Autodesk Inventor part; units mm, degrees
ref_plane "작업 평면1" through (-0.2823, -5.2823, -2.8) normal (0, 0, -1) x (0, 1, 0)
ref_plane "작업 평면2" through (1.8306, -3.1694, -7.8) normal (0, 0, -1) x (0, 1, 0)
ref_plane "YZ Plane" through (0, 0, 0) normal (1, 0, 0) x (0, 1, 0)
sketch "스케치1" plane through (0, 0, 0) normal (0, 0, 1) x (1, 0, 0)
  line L0 (5, 1.4434) -> (6.25, 0.7217)
  line L1 (6.25, 0.7217) -> (6.25, -0.7217)
  line L2 (6.25, -0.7217) -> (5, -1.4434)
  line L3 (5, -1.4434) -> (3.75, -0.7217)
  line L4 (3.75, -0.7217) -> (3.75, 0.7217)
  line L5 (3.75, 0.7217) -> (5, 1.4434)
  circle A0 centre (5, 0) radius 5
  circle A1 centre (5, 0) radius 5
  point P0 (0, 0)
ref_plane "작업 평면1" through (-0.2823, -5.2823, -2.8) normal (0, 0, -1) x (0, 1, 0)
extrude "돌출1" add sketch "스케치1" against normal up to surface (2.8 mm away)
sketch "스케치2" plane through (5, 0, -2.8) normal (0, 0, -1) x (-1, 0, 0)
  circle A0 centre (0, 0) radius 3
  circle A1 centre (0, 0) radius 2
  point P0 (5, 0)
ref_plane "작업 평면2" through (1.8306, -3.1694, -7.8) normal (0, 0, -1) x (0, 1, 0)
extrude "돌출2" add sketch "스케치2" along normal up to surface (5 mm away)
sketch "스케치3" plane through (5, 0, 0) normal (0, 0, 1) x (1, 0, 0)
  circle A0 centre (0, 0) radius 5
  line L0 (0, 1.4434) -> (1.25, 0.7217)
  line L1 (1.25, 0.7217) -> (1.25, -0.7217)
  line L2 (1.25, -0.7217) -> (0, -1.4434)
  line L3 (0, -1.4434) -> (-1.25, -0.7217)
  line L4 (-1.25, -0.7217) -> (-1.25, 0.7217)
  line L5 (-1.25, 0.7217) -> (0, 1.4434)
  circle A1 centre (0, 0) radius 2
  point P0 (-5, 0)
  dimension "d4" = 4
extrude "돌출3" cut sketch "스케치3" against normal through all contours L0 L1 L2 L3 L4 L5 | A1
chamfer "모따기1" distance 2.5 angle 45 1 edges at (3, 0, 0)
properties part number "Handmade tiered cover" material "LCP 플라스틱"
Can you work these out from the model? Positions are in its coordinate system, mm. A direction names the side the tool comes from. Give positions to 0.01 mm unless a question says otherwise; leave off trailing zeros. Loops run counter-clockwise (first coordinate to the right, second up) from the corner with the lowest first, then second, coordinate; pieces in that order, holes last. Notation, with made-up numbers: (61, 22.5) - (75, 22.5) arc R29 cw to (75, 58.5) - close; hole circle Ø11 at (34, -3). An arc over 180 degrees is marked (long way). Return JSON: item names as keys, results as strings.
1. If I drill on line 1 (Y direction, x = 5, z = -6.2); line 2 (Y direction, x = 6.25, z = -5.25); line 3 (X direction, y = 1.25, z = -0.25), over which ranges is the centre line in solid material (lowest first)?
Output values:
{"line 1": "y = -3 to -2, 2 to 3", "line 2": "y = -2.73 to -1.56, 1.56 to 2.73", "line 3": "x = 0.16 to 0.94, 9.06 to 9.84"}
2. I want a section at C-C on z = -7. Please give me the cut outline in (x, y).
Output values:
{"outline": "circle Ø6 at (5, 0); hole circle Ø4 at (5, 0)"}
3. For faces 1 (the face through (2.14, -0.9, -5.26)), 2 (the face through (4, -2, -7.8)), which set-ups out of +Z, -Z, +X, -X, +Y, -Y let a thin tool reach every point of the face, with its end or its side?
Output values:
{"face 1": "-Z", "face 2": "-Z, +X, -X, +Y, -Y"}
4. I'm going to push flat-ended pins straight in: pin 1 Ø3 at (y, z) = (-3, -5) entering from -X; pin 2 Ø1.5 at (x, z) = (6.5, -6.5) entering from +Y; pin 3 Ø3 at (x, z) = (6, -5) entering from +Y. Where does each tip first touch, or does it pass through?
Output values:
{"pin 1": "stops at x = 2.4", "pin 2": "stops at y = 2.9", "pin 3": "stops at y = 3"}
5. I want a section at B-B on y = 0. Please give me the cut outline in (x, z), and give its area (4 significant figures).
Output values:
{"outline": "(0, -2.8) - (2, -2.8) - (2, -7.8) - (3, -7.8) - (3, -2.5) - (0.5, 0) - (0, 0) - close; (7, -7.8) - (8, -7.8) - (8, -2.8) - (10, -2.8) - (10, 0) - (9.5, 0) - (7, -2.5) - close", "area": "20.55 mm²"}
6. We'd pull the mould along X, two halves only. Please class faces 3 (the face through (0, 0, -1)), 4 (the face through (4.9, -3.3, -2.8)), 5 (the face through (7.06, 0.65, -2.34)): +X half, -X half, draft (parallel to the pull), parting line (faces both ways), or undercut.
Output values:
{"face 3": "parting line", "face 4": "draft", "face 5": "undercut"}
7. I want a section at D-D on z = -0.75. Please give me the cut outline in (x, y), and give its area (3 significant figures).
Output values:
{"outline": "circle Ø10 at (5, 0); hole circle Ø7.5 at (5, 0)", "area": "34.4 mm²"}
8. I want a section at A-A on x = 5. Please give me the cut outline in (y, z), and give its area (4 significant figures).
Output values:
{"outline": "(-5, -2.8) - (-3, -2.8) - (-3, -7.8) - (-2, -7.8) - (-2, -2.5) - (-4.5, 0) - (-5, 0) - close; (2, -7.8) - (3, -7.8) - (3, -2.8) - (5, -2.8) - (5, 0) - (4.5, 0) - (2, -2.5) - close", "area": "20.55 mm²"}
